Here's the drawing with two shaded views (mm, measured from the low corner). I have some questions. Give positions to 0.01 mm unless a question says otherwise; leave off trailing zeros. Loops run counter-clockwise (first coordinate to the right, second up) from the corner with the lowest first, then second, coordinate; pieces in that order, holes last. Notation, with made-up numbers: (27, 16.5) -> (69, 16.5) arc R8 ccw to (69, 20.5) -> close; hole circle Ø10 at (25.5, 67). An arc over 180 degrees is marked (long way). Answer in a Markdown table with one row per item. Add a question column.
Item 1: If we section it at B-B (z = 135.5): Write out the boundary of the cut face in (x, y), then the cut area to 3 significant figures.
Item 2: If we section it at C-C (z = 24.5): Write out the boundary of the cut face in (x, y).
Item 3: If we section it at D-D (x = 24.5): Write out the boundary of the cut face in (y, z), then the cut area to 3 significant figures.
Item 4: For P1, Ø10, axis at x = 55, y = 3, coming from the +Z side; P2, Ø5, axis at x = 135.5, z = 24.5, coming from the +Y side; P3, Ø1.5, axis at x = 121.5, z = 47.5, coming from the +Y side; P4, Ø3, axis at x = 85, y = 2.5, coming from the +Z side, each with a flat end and sliding along its axis, tell me the tip position at first contact or that it passes through.
Item 5: If I drill on line 1 (X direction, y = 15.5, z = 135.5); line 2 (X direction, y = 9.5, z = 135.5); line 3 (Z direction, x = 24.5, y = 5.5), over which ranges is the centre line in solid material (lowest first)?
Item 6: If we section it at A-A (x = 80): Write out the boundary of the cut face in (y, z).
Item 7: We'd pull the mould along Z, two halves only. Please class the marked faces 1, 2 and 3: released by +Z, released by -Z, zero draft, split by the parting line, or undercut.
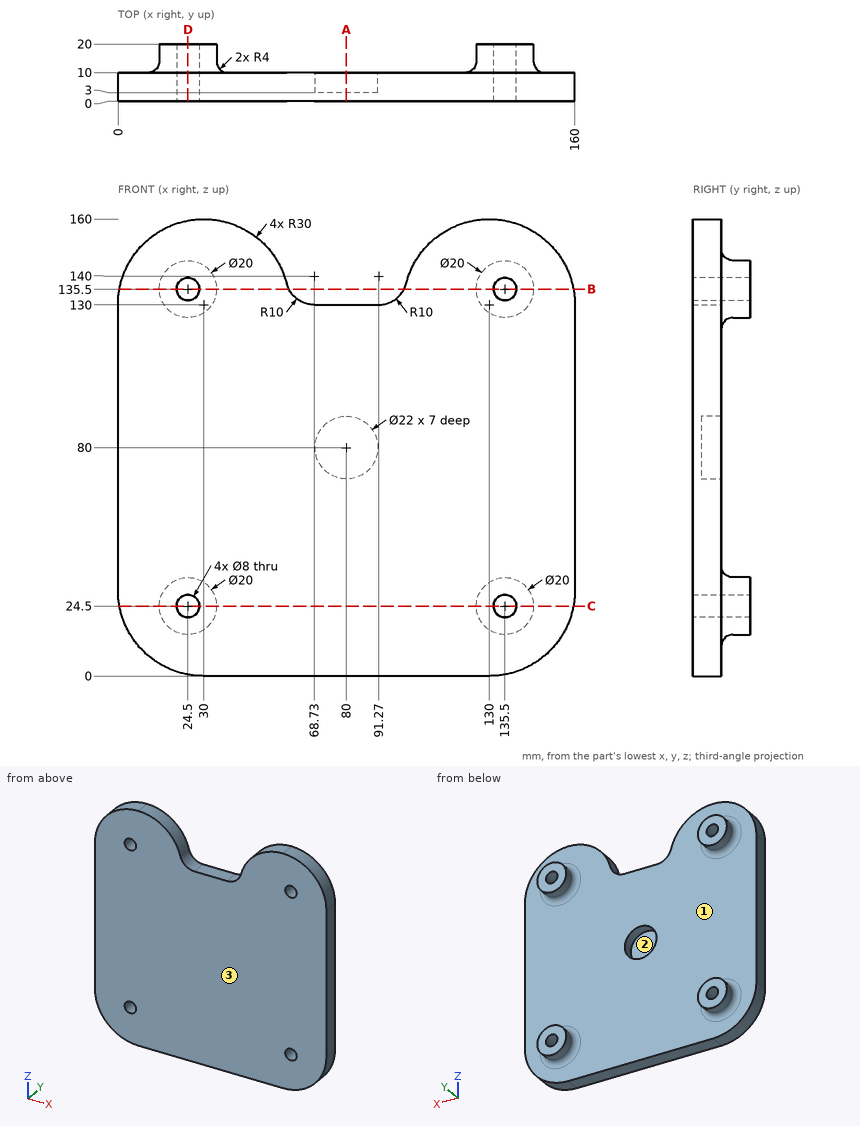
Recorded:
| question | item | result |
|---|---|---|
| 1 | outline | (0.51, 0) -> (20.5, 0) -> (20.5, 20) -> (14.5, 20) -> (14.5, 14) arc R4 cw to (10.5, 10) -> (0.51, 10) -> close; (28.5, 0) -> (59.8, 0) -> (59.8, 10) -> (38.5, 10) arc R4 cw to (34.5, 14) -> (34.5, 20) -> (28.5, 20) -> close; (100.2, 0) -> (131.5, 0) -> (131.5, 20) -> (125.5, 20) -> (125.5, 14) arc R4 cw to (121.5, 10) -> (100.2, 10) -> close; (139.5, 0) -> (159.49, 0) -> (159.49, 10) -> (149.5, 10) arc R4 cw to (145.5, 14) -> (145.5, 20) -> (139.5, 20) -> close |
| 1 | area | 1,280 mm^2 |
| 2 | outline | (0.51, 0) -> (20.5, 0) -> (20.5, 20) -> (14.5, 20) -> (14.5, 14) arc R4 cw to (10.5, 10) -> (0.51, 10) -> close; (28.5, 0) -> (131.5, 0) -> (131.5, 20) -> (125.5, 20) -> (125.5, 14) arc R4 cw to (121.5, 10) -> (38.5, 10) arc R4 cw to (34.5, 14) -> (34.5, 20) -> (28.5, 20) -> close; (139.5, 0) -> (159.49, 0) -> (159.49, 10) -> (149.5, 10) arc R4 cw to (145.5, 14) -> (145.5, 20) -> (139.5, 20) -> close |
| 3 | outline | (0, 0.51) -> (10, 0.51) -> (10, 10.5) arc R4 cw to (14, 14.5) -> (20, 14.5) -> (20, 20.5) -> (0, 20.5) -> close; (0, 28.5) -> (20, 28.5) -> (20, 34.5) -> (14, 34.5) arc R4 cw to (10, 38.5) -> (10, 121.5) arc R4 cw to (14, 125.5) -> (20, 125.5) -> (20, 131.5) -> (0, 131.5) -> close; (0, 139.5) -> (20, 139.5) -> (20, 145.5) -> (14, 145.5) arc R4 cw to (10, 149.5) -> (10, 159.49) -> (0, 159.49) -> close |
| 3 | area | 1,680 mm^2 |
| 4 | P1 | stops at z = 152.36 |
| 4 | P2 | passes through |
| 4 | P3 | stops at y = 10 |
| 4 | P4 | stops at z = 130 |
| 5 | line 1 | x = 14.5 to 20.5, 28.5 to 34.5, 125.5 to 131.5, 139.5 to 145.5 |
| 5 | line 2 | x = 0.51 to 20.5, 28.5 to 59.8, 100.2 to 131.5, 139.5 to 159.49 |
| 5 | line 3 | z = 0.51 to 20.5, 28.5 to 131.5, 139.5 to 159.49 |
| 6 | outline | (0, 0) -> (10, 0) -> (10, 69) -> (3, 69) -> (3, 91) -> (10, 91) -> (10, 130) -> (0, 130) -> close |
| 7 | face 1 | undercut |
| 7 | face 2 | undercut |
| 7 | face 3 | zero draft |
